Input: part model. Units: mm. Frame: model coordinates. A direction names the side the tool comes from. Round coordinates to 2 decimals unless told otherwise and drop trailing zeros. Loops run counter-clockwise (first coordinate to the right, second up) from the corner with the lowest first, then second, coordinate; pieces in that order, holes last. Notation, with made-up numbers: (16, 11) -> (73, 11) arc R22 cw to (73, 24) -> close; hole circle Ø11 at (-0.75, -27). An arc over 180 degrees is marked (long way). Answer in a Markdown table with one row per item. Add a question column.
Q1. Section A-A, the plane x = 18. Output: boundary loops of the cut face in (y, z).
Q2. Section C-C, the plane z = 7. Output: boundary loops of the cut face in (x, y).
Q3. Pin query (flat end, axial travel): pin 1 (0.7 mm diameter, centred on x = 28, y = 2, fed in from -Z); pin 2 (4 mm diameter, centred on x = -3, z = 2, fed in from +Y); pin 3 (2 mm diameter, centred on y = 36, z = 1, fed in from -X); pin 4 (5 mm diameter, centred on y = -11.5, z = 3.5, fed in from -X). Return the tip coordinate at first contact, or that it passes through.
Q4. Section B-B, the plane y = 34. Output: boundary loops of the cut face in (x, z), and give its area (3 significant figures).
Q5. Ray query, L1, parallel to X at y = -10.5, z = 4.5; L2, parallel to Y at x = -18, z = 0.8; L3, parallel to Z at x = -17.5, y = -15. Return the intervals inside material, ascending. Write a range as from..to.
Q6. Section D-D, the plane y = -20. Output: boundary loops of the cut face in (x, z).
Q7. Reachability of faces 4 (the face through (-23, 35, 1)), 5 (the face through (0, 31.5, 1)), 6 (the face through (-27.75, 0, 5)), 7 (the face through (25.6, 0, 1)), 8 (the face through (23, 35, 1)) from +Z, -Z, +X, -X, +Y, -Y: full face, straight path, thin tool, end or side. Return the list, or none.
Q8. Mould query, pull axis Y, two halves, no side actions, for faces 1 (the face through (13, 35, 1)), 2 (the face through (17.2, 35.5, 1.2)), 3 (the face through (-28, 31.5, 1)). Classes: pulls with the +Y half, pulls with the -Y half, needs draft (parallel to the pull), parting line crosses it, or undercut.
```python
from build123d import *

# Parameters (mm, degrees)
BOARD_SUPPORT_AND_LUGS_DEPTH = 2.5
PCB_EDGE_STOPS_START         = 2.5
SKETCH_PCB_EDGE_STOPS_W      = 2.5
SKETCH_PCB_EDGE_STOPS_H      = 56
PCB_EDGE_STOPS_DEPTH         = 6
BOARD_STRAP_SLOTS_START      = -1
SKETCH_BOARD_STRAP_SLOTS_W   = 2.8
SKETCH_BOARD_STRAP_SLOTS_H   = 10
BOARD_STRAP_SLOTS_DEPTH      = 4
EXTERNAL_M3_MOUNTS_START     = -1
SKETCH_EXTERNAL_M3_MOUNTS_R  = 1.7
EXTERNAL_M3_MOUNTS_DEPTH     = 5


with BuildPart() as part:
    # Sketch_Board_support_and_lugs → Board_support_and_lugs (new body)
    with BuildSketch(Plane.XY):
        Polygon((32, 31.5), (32, -31.5), (-32, -31.5), (-32, 31.5), (-23, 31.5), (-23, 38.5), (-13, 38.5), (-13, 31.5), (13, 31.5), (13, 38.5), (23, 38.5), (23, 31.5), align=None)
    extrude(amount=BOARD_SUPPORT_AND_LUGS_DEPTH)

    # Sketch_PCB_edge_stops → PCB_edge_stops (add)
    with BuildSketch(Plane.XY.offset(PCB_EDGE_STOPS_START)):
        with Locations((-29, 0)):
            Rectangle(SKETCH_PCB_EDGE_STOPS_W, SKETCH_PCB_EDGE_STOPS_H)
        with Locations((29, 0)):
            Rectangle(SKETCH_PCB_EDGE_STOPS_W, SKETCH_PCB_EDGE_STOPS_H)
    extrude(amount=PCB_EDGE_STOPS_DEPTH)

    # Sketch_Board_strap_slots → Board_strap_slots (cut)
    with BuildSketch(Plane.XY.offset(BOARD_STRAP_SLOTS_START)):
        with Locations((-27, 0)):
            Rectangle(SKETCH_BOARD_STRAP_SLOTS_W, SKETCH_BOARD_STRAP_SLOTS_H)
        with Locations((27, 0)):
            Rectangle(SKETCH_BOARD_STRAP_SLOTS_W, SKETCH_BOARD_STRAP_SLOTS_H)
    extrude(amount=BOARD_STRAP_SLOTS_DEPTH, mode=Mode.SUBTRACT)

    # Sketch_External_M3_mounts → External_M3_mounts (cut)
    with BuildSketch(Plane.XY.offset(EXTERNAL_M3_MOUNTS_START)):
        with Locations(Location((-18, 34, 0), (0, 0, 180))):
            Circle(SKETCH_EXTERNAL_M3_MOUNTS_R)
        with Locations(Location((18, 34, 0), (0, 0, 180))):
            Circle(SKETCH_EXTERNAL_M3_MOUNTS_R)
    extrude(amount=EXTERNAL_M3_MOUNTS_DEPTH, mode=Mode.SUBTRACT)


solid = part.part
```
Answer block:
| question | item | result |
|---|---|---|
| 1 | outline | (-31.5, 0) -> (32.3, 0) -> (32.3, 2.5) -> (-31.5, 2.5) -> close; (35.7, 0) -> (38.5, 0) -> (38.5, 2.5) -> (35.7, 2.5) -> close |
| 2 | outline | (-30.25, -28) -> (-27.75, -28) -> (-27.75, 28) -> (-30.25, 28) -> close; (27.75, -28) -> (30.25, -28) -> (30.25, 28) -> (27.75, 28) -> close |
| 3 | pin 1 | z = 3 |
| 3 | pin 2 | y = 31.5 |
| 3 | pin 3 | x = -23 |
| 3 | pin 4 | x = -32 |
| 4 | outline | (-23, 0) -> (-19.7, 0) -> (-19.7, 2.5) -> (-23, 2.5) -> close; (-16.3, 0) -> (-13, 0) -> (-13, 2.5) -> (-16.3, 2.5) -> close; (13, 0) -> (16.3, 0) -> (16.3, 2.5) -> (13, 2.5) -> close; (19.7, 0) -> (23, 0) -> (23, 2.5) -> (19.7, 2.5) -> close |
| 4 | area | 33.0 mm^2 |
| 5 | L1 | -30.25..-27.75, 27.75..30.25 |
| 5 | L2 | -31.5..32.3, 35.7..38.5 |
| 5 | L3 | 0..2.5 |
| 6 | outline | (-32, 0) -> (32, 0) -> (32, 2.5) -> (30.25, 2.5) -> (30.25, 8.5) -> (27.75, 8.5) -> (27.75, 2.5) -> (-27.75, 2.5) -> (-27.75, 8.5) -> (-30.25, 8.5) -> (-30.25, 2.5) -> (-32, 2.5) -> close |
| 7 | face 4 | +Z, -Z, -X, +Y |
| 7 | face 5 | +Z, -Z, +Y |
| 7 | face 6 | +Z, +Y, -Y |
| 7 | face 7 | +Z, -Z |
| 7 | face 8 | +Z, -Z, +X, +Y |
| 8 | face 1 | needs draft |
| 8 | face 2 | undercut |
| 8 | face 3 | pulls with the +Y half |
